from build123d import *

# Parameters (mm, degrees)
SKETCH1_R           = 1.7272
BOSS_EXTRUDE1_DEPTH = 3.2004
SKETCH2_W           = 9.525
SKETCH2_H           = 25.4
CUT_EXTRUDE1_DEPTH  = 3.2004
SKETCH3_R           = 1.1303
CUT_EXTRUDE2_DEPTH  = 3.2004
FILLET1_R           = 2.54
SKETCH4_R           = 1.02489
CUT_EXTRUDE3_DEPTH  = 3.2004


with BuildPart() as part:
    # Sketch1 → Boss-Extrude1 (new body)
    with BuildSketch(Plane(origin=(0, 0, 0), x_dir=(1, 0, 0), z_dir=(0, 1, 0))):
        Polygon((0, 136.525), (0, 0), (107.315, 0), (107.315, 120.4468), (81.915, 120.4468), (81.915, 136.525), align=None)
        with Locations((10.795, 128.8415)):
            Circle(SKETCH1_R, mode=Mode.SUBTRACT)
        with Locations((96.52, 7.6835)):
            Circle(SKETCH1_R, mode=Mode.SUBTRACT)
        with Locations((10.795, 7.6835)):
            Circle(SKETCH1_R, mode=Mode.SUBTRACT)
        with Locations((74.295, 128.8415)):
            Circle(SKETCH1_R, mode=Mode.SUBTRACT)
    extrude(amount=BOSS_EXTRUDE1_DEPTH)

    # Sketch2 → Cut-Extrude1 (cut)
    with BuildSketch(Plane(origin=(0, 3.2004, 0), x_dir=(1, 0, 0), z_dir=(0, 1, 0))):
        with Locations((24.4475, 103.505)):
            Rectangle(SKETCH2_W, SKETCH2_H)
        with BuildLine():
            Line((0, 116.330365836), (0, 90.679634164))
            ThreePointArc((0, 90.679634164), (12.825365836, 103.505), (0, 116.330365836))
        make_face()
    extrude(amount=-CUT_EXTRUDE1_DEPTH, mode=Mode.SUBTRACT)

    # Sketch3 → Cut-Extrude2 (cut)
    with BuildSketch(Plane(origin=(0, 3.2004, 0), x_dir=(1, 0, 0), z_dir=(0, 1, 0))):
        with Locations((92.312807391, 101.2825)):
            Circle(SKETCH3_R)
        with Locations((92.312807391, 35.2425)):
            Circle(SKETCH3_R)
        with Locations((16.112807391, 35.2425)):
            Circle(SKETCH3_R)
        with Locations((16.112807391, 101.2825)):
            Circle(SKETCH3_R)
    extrude(amount=-CUT_EXTRUDE2_DEPTH, mode=Mode.SUBTRACT)

    # Fillet1
    fillet1_edges = [part.edges().sort_by_distance(p)[0] for p in [
        (0, 1.6002, 0),
        (0, 1.6002, -136.525),
        (81.915, 1.6002, -136.525),
        (107.315, 1.6002, -120.4468),
        (107.315, 1.6002, 0),
        (0, 1.6002, -90.679634164),
        (0, 1.6002, -116.330365836),
    ]]
    fillet(fillet1_edges, radius=FILLET1_R)

    # Sketch4 → Cut-Extrude3 (cut)
    with BuildSketch(Plane(origin=(0, 3.2004, 0), x_dir=(1, 0, 0), z_dir=(0, 1, 0))):
        with Locations((64.6575, 75.7625)):
            Circle(SKETCH4_R)
        with Locations((64.6575, 60.7625)):
            Circle(SKETCH4_R)
        with Locations((42.6575, 75.7625)):
            Circle(SKETCH4_R)
        with Locations((42.6575, 60.7625)):
            Circle(SKETCH4_R)
    extrude(amount=-CUT_EXTRUDE3_DEPTH, mode=Mode.SUBTRACT)


solid = part.part
Source: CAD feature listing. Evaluate the final solid. Frame: model axes, mm. A direction names the side the tool comes from. Coordinates: 2 decimals unless noted, no trailing zeros. Loops run counter-clockwise (first coordinate to the right, second up) from the corner with the lowest first, then second, coordinate; pieces in that order, holes last. Notation, with made-up numbers: (17, 36.25) -> (43, 36.25) arc R20 ccw to (43, 68.25) -> close; hole circle Ø4 at (46, -22.75). An arc over 180 degrees is marked (long way). Answer in a Markdown table with one row per item. Add a question column.
Q1. Section C-C on y = 2.65. Give the number of separate pieces and of enclosed holes in the cut face, and give its area (3 significant figures).
Q2. Section A-A on x = 96.52. Return the cut outline in (y, z).
Q3. Section B-B on x = 27. Return the cut outline in (y, z) (3 decimals).
Q4. Contact query for flat-ended pins moving along their axis: pin 1 Ø2.5 at (x, z) = (16.11, -101.28) entering from -Y; pin 2 Ø1 at (x, y) = (85.5, 2) entering from -Z. Output: stop coordinate, or through.
Q5. Reachability of faces 1 (the face through (53, 0, -69)), 2 (the face through (29.21, 2, -103)), 3 (the face through (81.915, 2, -127)) from +Z, -Z, +X, -X, +Y, -Y: full face, straight path, thin tool, end or side. Return the list, or none.
Q6. Ray query, line 1 along Z through (x, y) = (42.5, 2.35) (3 decimals); line 2 along Z through (x, y) = (21.5, 0.8) (3 decimals); line 3 along Z through (x, y) = (74.5, 2.2) (1 decimal). Return the intervals inside material, ascending.
Q7. Pull-direction query (Z, two-part tool) for faces 4 (the face through (24, 2, -90.805)), 5 (the face through (53, 3.2, -69)), 6 (the face through (94, 2, -120.447)); classes: pulls with the +Z half, pulls with the -Z half, needs draft (parallel to the pull), parting line crosses it, or undercut.
Computed values:
| question | item | result |
|---|---|---|
| 1 | separate pieces | 1 |
| 1 | enclosed holes | 13 |
| 1 | area | 13,700 mm^2 |
| 2 | outline | (0, -120.45) -> (3.2, -120.45) -> (3.2, -9.41) -> (0, -9.41) -> close; (0, -5.96) -> (3.2, -5.96) -> (3.2, 0) -> (0, 0) -> close |
| 3 | outline | (0, -136.525) -> (3.2, -136.525) -> (3.2, -116.205) -> (0, -116.205) -> close; (0, -90.805) -> (3.2, -90.805) -> (3.2, 0) -> (0, 0) -> close |
| 4 | pin 1 | stops at y = 0 |
| 4 | pin 2 | stops at z = -120.45 |
| 5 | face 1 | +Z, -Z, +X, -X, -Y |
| 5 | face 2 | +Y, -Y |
| 5 | face 3 | -Z, +X, +Y, -Y |
| 6 | line 1 | z = -136.525 to -76.775, -74.75 to -61.775, -59.75 to 0 |
| 6 | line 2 | z = -136.525 to -116.205, -90.805 to 0 |
| 6 | line 3 | z = -136.5 to -130.6, -127.1 to 0 |
| 7 | face 4 | undercut |
| 7 | face 5 | needs draft |
| 7 | face 6 | pulls with the -Z half |
